The figure shows three views and two pictorial views of one solid part (mm, origin at its lowest corner). Answer the questions. Give positions to 0.01 mm unless a question says otherwise; leave off trailing zeros. Order: outer loops, then holes, each group sorted by start corner. A loop starts at its lowest first (then second) coordinate and runs counter-clockwise, first axis right, second up. Notation, with made-up numbers: (80, 68) - (100, 68) arc R6 ccw to (100, 77) - close; hole circle Ø6 at (64.25, 39.25). An arc over 180 degrees is marked (long way). Answer as CSV lines item,"result". Start each with the question number.
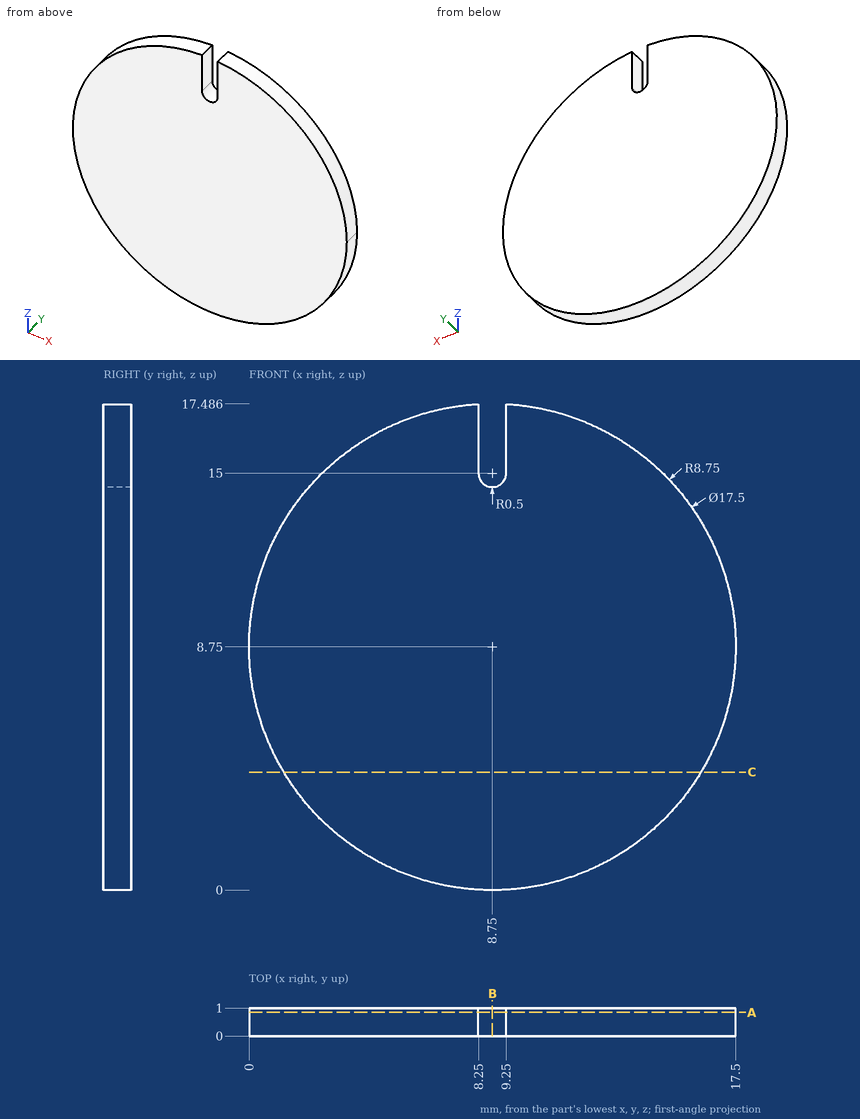
(1) Straight lines are drawn through the part: line 1 (X direction, y = 0.5, z = 8.5); line 2 (X direction, y = 0.7, z = 16); line 3 (X direction, y = 0.85, z = 3.25) (1 decimal). For each, find the intervals that lie inside material, in ascending order. Write a range as [from, to].
(2) Section B-B, the plane x = 8.75 is taken. Write down the section's boundary in (y, z).
(3) Section C-C, the plane z = 4.25 is taken. Write down the section's boundary in (x, y).
(4) Section A-A, the plane y = 0.85 is taken. Write down the section's boundary in (x, z), and give its area (3 significant figures).
Checks:
1,line 1,"x = [0, 17.5]"
1,line 2,"x = [3.85, 8.25], [9.25, 13.65]"
1,line 3,"x = [1.9, 15.6]"
2,outline,"(0, 0) - (1, 0) - (1, 14.5) - (0, 14.5) - close"
3,outline,"(1.25, 0) - (16.25, 0) - (16.25, 1) - (1.25, 1) - close"
4,outline,"(8.25, 15) - (8.25, 17.49) arc R8.75 ccw (long way) to (9.25, 17.49) - (9.25, 15) arc R0.5 cw to start"
4,area,"238 mm²"
